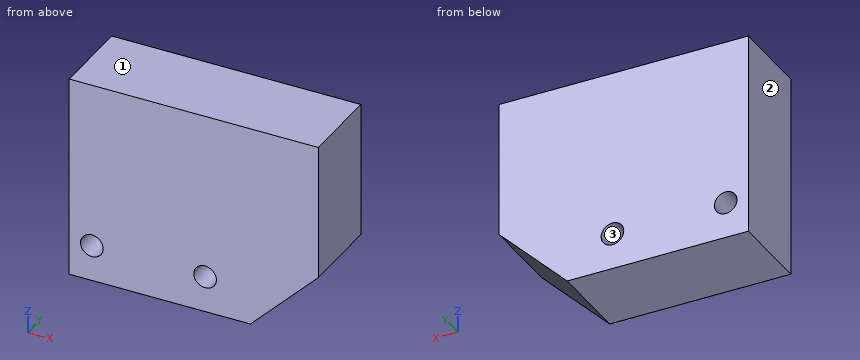
```python
from build123d import *

# Parameters (mm, degrees)
F0_W     = 55
F0_H     = 45
F1_DEPTH = 18
F3_SIZE  = 15
F4_D     = 5


with BuildPart() as f1:
    # F0 (on Front) → F1 (new body)
    with BuildSketch(Plane.XZ):
        with Locations((27.5, 22.5)):
            Rectangle(F0_W, F0_H)
    extrude(amount=F1_DEPTH)

    # F3
    f3_edges = [f1.edges().sort_by_distance(p)[0] for p in [
        (55, -9, 0),
    ]]
    chamfer(f3_edges, length=F3_SIZE)

    # F4 (through all)
    with Locations(Plane.XZ.offset(18)):
        with Locations((30, 8), (5, 8)):
            Hole(F4_D / 2)


solid = f1.part
```
Read the model definition and answer for the solid it produces. Units are mm, in the model's axes. Face numbers are marked on the shaded views. Coordinates: 2 decimals unless noted, no trailing zeros. Order: outer loops, then holes, each group sorted by start corner. A loop starts at its lowest first (then second) coordinate and runs counter-clockwise, first axis right, second up. Notation, with made-up numbers: (88, 1) - (126, 1) arc R18 ccw to (126, 10) - close; hole circle Ø10 at (58, 17.25). An arc over 180 degrees is marked (long way). Answer as a JSON object with one key per item and string values. Group by question number.
Item 1: A flat-ended cylindrical pin translates along its axis: P1, Ø5, axis at x = 14, z = 28.5, coming from the +Y side. Find the tip coordinate at first contact, or state that the pin passes through.
Item 2: Section D-D (x = 29.5) is taken. Give the vertices of the cut face in (y, z).
Item 3: Consider probe 1 along Z at (x, y) = (5, -4.25); probe 2 along Z at (x, y) = (4, -11); probe 3 along X at (y, z) = (-5, 9.5). Determine where each line is inside the solid, lowest interval first. Write a range as from..to.
Item 4: Section A-A (x = 5) is taken. Give the vertices of the cut face in (y, z).
Item 5: Section C-C (y = -11.75) is taken. Give the vertices of the cut face in (x, z), plus the area to 3 significant figures.
Item 6: The mould has two halves that part along Z. Classify the marked faces 1, 2 and 3: +Z half, -Z half, draft (parallel to the pull), parting line (faces both ways), or undercut.
Item 7: Section B-B (z = 8) is taken. Give the vertices of the cut face in (x, y), plus the area to 3 significant figures.
Results are:
{
 "1": {"P1": "stops at y = 0"},
 "2": {"outline": "(-18, 0) - (0, 0) - (0, 5.55) - (-18, 5.55) - close; (-18, 10.45) - (0, 10.45) - (0, 45) - (-18, 45) - close"},
 "3": {"probe 1": "z = 0..5.5, 10.5..45", "probe 2": "z = 0..5.71, 10.29..45", "probe 3": "x = 0..3, 7..28, 32..49.5"},
 "4": {"outline": "(-18, 0) - (0, 0) - (0, 5.5) - (-18, 5.5) - close; (-18, 10.5) - (0, 10.5) - (0, 45) - (-18, 45) - close"},
 "5": {"outline": "(0, 0) - (40, 0) - (55, 15) - (55, 45) - (0, 45) - close; hole circle Ø5 at (5, 8); hole circle Ø5 at (30, 8)", "area": "2,320 mm^2"},
 "6": {"face 1": "+Z half", "face 2": "draft", "face 3": "undercut"},
 "7": {"outline": "(0, -18) - (2.5, -18) - (2.5, 0) - (0, 0) - close; (7.5, -18) - (27.5, -18) - (27.5, 0) - (7.5, 0) - close; (32.5, -18) - (48, -18) - (48, 0) - (32.5, 0) - close", "area": "684 mm^2"}
}
